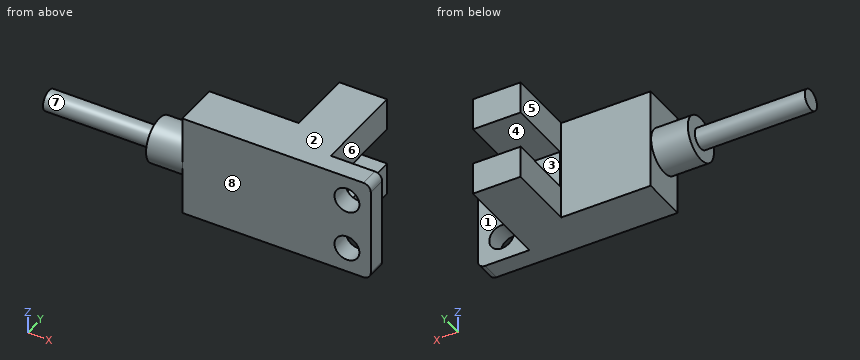
from build123d import *

# Parameters (mm, degrees)
BOSS_EXTRU_1_DEPTH           = 6.9
ENL_V_MAT_EXTRU_1_DEPTH      = 23.946949688
ENL_V_MAT_EXTRU_1_DEPTH_BACK = 23.946949688
ESQUISSE2_W                  = 5
ESQUISSE2_H                  = 9
D_GAGEMENT_M31_D             = 3.4
ESQUISSE5_R                  = 3
BOSS_EXTRU_2_DEPTH           = 5
ESQUISSE6_R                  = 1.4
BOSS_EXTRU_3_DEPTH           = 15
CONG_1_R                     = 1


with BuildPart() as part:
    # Esquisse1 → Boss.-Extru.1 (new, symmetric)
    with BuildSketch(Plane.XY):
        Polygon((-15.45, 0), (10.25, 0), (10.25, 2.6), (3.25, 2.6), (3.25, 15.5), (-3.25, 15.5), (-3.25, 6.2), (-15.45, 6.2), align=None)
    extrude(amount=BOSS_EXTRU_1_DEPTH, both=True)

    # Esquisse2 → Enlèv. mat.-Extru.1 (cut, two sides: drawn at the far end of the back side and taken through both)
    with BuildSketch(Plane(origin=(0, 0, 0), x_dir=(0, 0, -1), z_dir=(1, 0, 0)).offset(-ENL_V_MAT_EXTRU_1_DEPTH_BACK)):
        with Locations((0, 11)):
            Rectangle(ESQUISSE2_W, ESQUISSE2_H)
    extrude(amount=ENL_V_MAT_EXTRU_1_DEPTH + ENL_V_MAT_EXTRU_1_DEPTH_BACK, mode=Mode.SUBTRACT)

    # Dégagement M31 (through all)
    with Locations(Plane(origin=(0, 2.6, 0), x_dir=(1, 0, 0), z_dir=(0, 1, 0))):
        with Locations((7, 3.5), (7, -3.5)):
            Hole(D_GAGEMENT_M31_D / 2)

    # Esquisse5 → Boss.-Extru.2 (add)
    with BuildSketch(Plane.ZY.offset(15.45)):
        with Locations((0, 3.1)):
            Circle(ESQUISSE5_R)
    extrude(amount=BOSS_EXTRU_2_DEPTH)

    # Esquisse6 → Boss.-Extru.3 (add)
    with BuildSketch(Plane.ZY.offset(20.45)):
        with Locations((0, 3.1)):
            Circle(ESQUISSE6_R)
    extrude(amount=BOSS_EXTRU_3_DEPTH)

    # Congé1
    cong_1_edges = [part.edges().sort_by_distance(p)[0] for p in [
        (10.25, 1.3, -6.9),
        (10.25, 1.3, 6.9),
    ]]
    fillet(cong_1_edges, radius=CONG_1_R)


solid = part.part
Input: part model. Units: mm. Frame: model coordinates. Face numbers are marked on the shaded views. A direction names the side the tool comes from. Round coordinates to 2 decimals unless told otherwise and drop trailing zeros. Order: outer loops, then holes, each group sorted by start corner. A loop starts at its lowest first (then second) coordinate and runs counter-clockwise, first axis right, second up. Notation, with made-up numbers: (-19.5, 68.25) - (21.5, 68.25) arc R4 ccw to (21.5, 75.25) - close; hole circle Ø6 at (74.5, 45). An arc over 180 degrees is marked (long way). Answer as a JSON object with one key per item and string values. Group by question number.
(1) Pin query (flat end, axial travel): P1, Ø7.5, axis at y = 11, z = -3, coming from the -X side; P2, Ø5, axis at x = -21.5, z = 2, coming from the -Y side; P3, Ø1.5, axis at x = 0, z = 1, coming from the +Y side; P4, Ø2, axis at x = 7, z = -3.5, coming from the -Y side. Return the tip coordinate at first contact, or that it passes through.
(2) Cut plane B-B (z = -3.5). Return loops of the section in (x, y).
(3) Cut plane C-C (y = 7). Return loops of the section in (x, z).
(4) Cut plane D-D (z = 0). Return loops of the section in (x, y), then the cut area to 3 significant figures.
(5) Reachability of the marked faces 4, 5, 6, 7 and 8 from +Z, -Z, +X, -X, +Y, -Y: full face, straight path, thin tool, end or side. Return the list, or none.
(6) Material intervals for probe 1 along Z at (x, y) = (7, 1.25); probe 2 along Y at (x, z) = (-12.5, -2.75); probe 3 along X at (y, z) = (9, -3), sorted ascending. Write a range as from..to.
(7) Cut plane A-A (x = 7). Return loops of the section in (y, z), then the cut area to 3 significant figures.
(8) Draft query along Z for the marked faces 1, 2 and 3. Return one class per face: released by +Z, released by -Z, zero draft, split by the parting line, or undercut.
Here are the results:
{
 "1": {"P1": "stops at x = -3.25", "P2": "stops at y = 0.1", "P3": "stops at y = 6.5", "P4": "passes through"},
 "2": {"outline": "(-15.45, 0) - (5.3, 0) - (5.3, 2.6) - (3.25, 2.6) - (3.25, 15.5) - (-3.25, 15.5) - (-3.25, 6.2) - (-15.45, 6.2) - close; (8.7, 0) - (10.25, 0) - (10.25, 2.6) - (8.7, 2.6) - close"},
 "3": {"outline": "(-3.25, -6.9) - (3.25, -6.9) - (3.25, -2.5) - (-3.25, -2.5) - close; (-3.25, 2.5) - (3.25, 2.5) - (3.25, 6.9) - (-3.25, 6.9) - close"},
 "4": {"outline": "(-35.45, 1.7) - (-20.45, 1.7) - (-20.45, 0.1) - (-15.45, 0.1) - (-15.45, 0) - (10.25, 0) - (10.25, 2.6) - (3.25, 2.6) - (3.25, 6.5) - (-3.25, 6.5) - (-3.25, 6.2) - (-15.45, 6.2) - (-15.45, 6.1) - (-20.45, 6.1) - (-20.45, 4.5) - (-35.45, 4.5) - close", "area": "208 mm^2"},
 "5": {"face 4": "+X, -X, +Y", "face 5": "+Z, -Z, -X, +Y", "face 6": "+Z, -Z, +X, +Y", "face 7": "-X", "face 8": "+Z, -Z, +X, -X, -Y"},
 "6": {"probe 1": "z = -6.9..-5.2, -1.8..1.8, 5.2..6.9", "probe 2": "y = 0..6.2", "probe 3": "x = -3.25..3.25"},
 "7": {"outline": "(0, -6.9) - (2.6, -6.9) - (2.6, -5.2) - (0, -5.2) - close; (0, -1.8) - (2.6, -1.8) - (2.6, 1.8) - (0, 1.8) - close; (0, 5.2) - (2.6, 5.2) - (2.6, 6.9) - (0, 6.9) - close", "area": "18.2 mm^2"},
 "8": {"face 1": "zero draft", "face 2": "released by +Z", "face 3": "undercut"}
}
